The listing builds one solid part. Answer for the finished solid, in the listing's coordinates (mm). Coordinates: 2 decimals unless noted, no trailing zeros. Write each loop counter-clockwise with the first axis right and the second up, starting at its lowest first coordinate (ties: lowest second). Pieces come first, ordered by that corner, then holes.
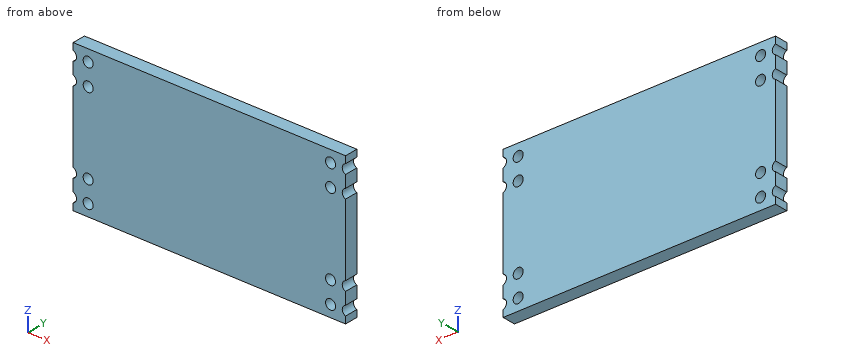
from build123d import *

# Parameters (mm, degrees)
SKETCH1_W                       = 32.7
SKETCH1_H                       = 17.72
MAIN_BODY_DEPTH                 = 1.6
SKETCH2_R                       = 0.6
SOLDERED_CONNECTION_HOLES_DEPTH = 19.664996651
LPATTERN1_COUNT                 = 2
LPATTERN1_PITCH                 = 2
MIRROR1_COPY_1_SKETCH_R         = 0.6
MIRROR1_COPY_1_DEPTH            = 19.664996651
MIRROR2_COPY_1_SKETCH_R         = 0.6
MIRROR2_COPY_1_DEPTH            = 19.664996651
MIRROR2_COPY_2_SKETCH_R         = 0.6
MIRROR2_COPY_2_DEPTH            = 19.664996651
MIRROR2_COPY_3_SKETCH_R         = 0.6
MIRROR2_COPY_3_DEPTH            = 19.664996651


with BuildPart() as part:
    # Sketch1 → MAIN BODY (new body)
    with BuildSketch(Plane(origin=(0, 0, 0), x_dir=(1, 0, 0), z_dir=(0, 1, 0))):
        Rectangle(SKETCH1_W, SKETCH1_H)
    extrude(amount=MAIN_BODY_DEPTH)

    # Sketch2 → SOLDERED CONNECTION HOLES (cut, through all)
    with BuildSketch(Plane(origin=(0, 1.6, 0), x_dir=(1, 0, 0), z_dir=(0, 1, 0))):
        with Locations(Location((-14.55, 7.46, 0), (0, 0, 270))):
            Circle(SKETCH2_R)
        with Locations(Location((-14.55, 4.86, 0), (0, 0, 270))):
            Circle(SKETCH2_R)
    soldered_connection_holes = extrude(amount=-SOLDERED_CONNECTION_HOLES_DEPTH, mode=Mode.SUBTRACT)

    # LPattern1: SOLDERED CONNECTION HOLES ×2
    with Locations(*[(-i * LPATTERN1_PITCH, 0, 0) for i in range(1, LPATTERN1_COUNT)]):
        add(soldered_connection_holes, mode=Mode.SUBTRACT)

    # Mirror1: SOLDERED CONNECTION HOLES across plane
    add(soldered_connection_holes.mirror(Plane(origin=(0, 0, 0), x_dir=(0, 0, 1), z_dir=(1, 0, 0))), mode=Mode.SUBTRACT)

    # Mirror1 copy 1 sketch → Mirror1 copy 1 (cut, through all)
    with BuildSketch(Plane(origin=(2, 1.6, 0), x_dir=(-1, 0, 0), z_dir=(0, 1, 0))):
        with Locations((-14.55, -7.46)):
            Circle(MIRROR1_COPY_1_SKETCH_R)
        with Locations((-14.55, -4.86)):
            Circle(MIRROR1_COPY_1_SKETCH_R)
    extrude(amount=-MIRROR1_COPY_1_DEPTH, mode=Mode.SUBTRACT)

    # Mirror2: SOLDERED CONNECTION HOLES across plane
    add(soldered_connection_holes.mirror(Plane.XY), mode=Mode.SUBTRACT)

    # Mirror2 copy 1 sketch → Mirror2 copy 1 (cut, through all)
    with BuildSketch(Plane(origin=(-2, 1.6, 0), x_dir=(1, 0, 0), z_dir=(0, 1, 0))):
        with Locations((-14.55, -7.46)):
            Circle(MIRROR2_COPY_1_SKETCH_R)
        with Locations((-14.55, -4.86)):
            Circle(MIRROR2_COPY_1_SKETCH_R)
    extrude(amount=-MIRROR2_COPY_1_DEPTH, mode=Mode.SUBTRACT)

    # Mirror2 copy 2 sketch → Mirror2 copy 2 (cut, through all)
    with BuildSketch(Plane(origin=(0, 1.6, 0), x_dir=(-1, 0, 0), z_dir=(0, 1, 0))):
        with Locations(Location((-14.55, 7.46, 0), (0, 0, 270))):
            Circle(MIRROR2_COPY_2_SKETCH_R)
        with Locations(Location((-14.55, 4.86, 0), (0, 0, 270))):
            Circle(MIRROR2_COPY_2_SKETCH_R)
    extrude(amount=-MIRROR2_COPY_2_DEPTH, mode=Mode.SUBTRACT)

    # Mirror2 copy 3 sketch → Mirror2 copy 3 (cut, through all)
    with BuildSketch(Plane(origin=(2, 1.6, 0), x_dir=(-1, 0, 0), z_dir=(0, 1, 0))):
        with Locations(Location((-14.55, 7.46, 0), (0, 0, 270))):
            Circle(MIRROR2_COPY_3_SKETCH_R)
        with Locations(Location((-14.55, 4.86, 0), (0, 0, 270))):
            Circle(MIRROR2_COPY_3_SKETCH_R)
    extrude(amount=-MIRROR2_COPY_3_DEPTH, mode=Mode.SUBTRACT)


solid = part.part
Q1. Find the intervals of material crossed by probe 1 along Z at (x, y) = (14.55, 0.7); probe 2 along X at (y, z) = (0.6, 7.46); probe 3 along X at (y, z) = (0.25, 4.5), in increasing order.
Answers below:
probe 1: z = -8.86 to -8.06, -6.86 to -5.46, -4.26 to 4.26, 5.46 to 6.86, 8.06 to 8.86
probe 2: x = -15.95 to -15.15, -13.95 to 13.95, 15.15 to 15.95
probe 3: x = -16.07 to -15.03, -14.07 to 14.07, 15.03 to 16.07
Q2. The part is cut by section B-B, the plane z = -7.46. Write down the section's boundary in (x, y), then the cut area to 3 significant figures.
Answers below:
outline: (-15.95, 0) - (-15.15, 0) - (-15.15, 1.6) - (-15.95, 1.6) - close; (-13.95, 0) - (13.95, 0) - (13.95, 1.6) - (-13.95, 1.6) - close; (15.15, 0) - (15.95, 0) - (15.95, 1.6) - (15.15, 1.6) - close
area: 47.2 mm2
Q3. The part is cut by section C-C, the plane y = 0.7. State how many separate pieces and enclosed holes the cut face has, then the cut area to 3 significant figures.
Answers below:
separate pieces: 1
enclosed holes: 8
area: 568 mm2
Q4. The part is cut by section A-A, the plane x = 14.55. Write down the section's boundary in (y, z), then the cut area to 3 significant figures.
Answers below:
outline: (0, -8.86) - (1.6, -8.86) - (1.6, -8.06) - (0, -8.06) - close; (0, -6.86) - (1.6, -6.86) - (1.6, -5.46) - (0, -5.46) - close; (0, -4.26) - (1.6, -4.26) - (1.6, 4.26) - (0, 4.26) - close; (0, 5.46) - (1.6, 5.46) - (1.6, 6.86) - (0, 6.86) - close; (0, 8.06) - (1.6, 8.06) - (1.6, 8.86) - (0, 8.86) - close
area: 20.7 mm2
